Can you work these out from the model? Positions are in its coordinate system, mm. A direction names the side the tool comes from. Round coordinates to 2 decimals unless told otherwise and drop trailing zeros. Loops run counter-clockwise (first coordinate to the right, second up) from the corner with the lowest first, then second, coordinate; pieces in that order, holes last. Notation, with made-up numbers: M 75.25,17 L 111.25,17 A17 cw 111.25,43 Z; hole C 70.5,42.25 d7. An arc over 180 degrees is marked long. Answer as CSV lines item,"result".
from build123d import *

# Parameters (mm, degrees)
BOSS_EXTRUDE1_DEPTH     = 6
CUT_EXTRUDE1_DEPTH      = 33.32645975048922
CUT_EXTRUDE1_DEPTH_BACK = 33.32645975048922
SKETCH3_R               = 1.7500000000000002
SKETCH3_R_2             = 1.7499999999999998
SKETCH6_R               = 3.2500000000000004
SKETCH6_R_2             = 3.25
CUT_EXTRUDE2_DEPTH      = 3.5
SKETCH7_W               = 11.699999999999998
SKETCH7_H               = 27.786688839798195
BOSS_EXTRUDE2_DEPTH     = 6
SKETCH8_W               = 11.699999999999998
SKETCH8_H               = 27.786688839798195
CUT_EXTRUDE3_DEPTH      = 2
FILLET1_R               = 2
FILLET2_R               = 2
FILLET3_R               = 2
CUT_EXTRUDE4_DEPTH      = 52.48495646180262
CUT_EXTRUDE4_DEPTH_BACK = 52.48495646180262
CUT_EXTRUDE5_DEPTH      = 52.48495646180262
CUT_EXTRUDE5_DEPTH_BACK = 2
FILLET4_R               = 2
FILLET5_R               = 2


with BuildPart() as part:
    # Sketch2 → Boss-Extrude1 (new body)
    with BuildSketch(Plane.XY):
        Polygon((-27.999999999999996, 15), (1.84e-15, 15), (0, 0), (-27.999999999999996, 0), align=None)
    extrude(amount=BOSS_EXTRUDE1_DEPTH)

    # Sketch3 → Cut-Extrude1 (cut, two sides: drawn at the far end of the back side and taken through both)
    with BuildSketch(Plane.XY.offset(6).offset(-CUT_EXTRUDE1_DEPTH_BACK)):
        with Locations((-21.5, 4.999999999999999)):
            Circle(SKETCH3_R)
        with Locations((-6.5, 4.999999999999999)):
            Circle(SKETCH3_R_2)
    extrude(amount=CUT_EXTRUDE1_DEPTH + CUT_EXTRUDE1_DEPTH_BACK, mode=Mode.SUBTRACT)

    # Sketch6 → Cut-Extrude2 (cut)
    with BuildSketch(Plane.XY.offset(6)):
        with Locations((-21.5, 4.999999999999999)):
            Circle(SKETCH6_R)
        with Locations((-6.500000000000001, 4.999999999999999)):
            Circle(SKETCH6_R_2)
    extrude(amount=-CUT_EXTRUDE2_DEPTH, mode=Mode.SUBTRACT)

    # Sketch7 → Boss-Extrude2 (add)
    with BuildSketch(Plane(origin=(0, 0, 0), x_dir=(-1, 0, 0), z_dir=(0, 0, -1))):
        with Locations((14, 28.893344419899098)):
            Rectangle(SKETCH7_W, SKETCH7_H)
    extrude(amount=-BOSS_EXTRUDE2_DEPTH)

    # Sketch8 → Cut-Extrude3 (cut)
    with BuildSketch(Plane(origin=(0, 0, 0), x_dir=(-1, 0, 0), z_dir=(0, 0, -1))):
        with Locations((14, 28.893344419899098)):
            Rectangle(SKETCH8_W, SKETCH8_H)
    extrude(amount=-CUT_EXTRUDE3_DEPTH, mode=Mode.SUBTRACT)

    # Fillet1
    fillet1_edges = [part.edges().sort_by_distance(p)[0] for p in [
        (-14, 15, 2),
    ]]
    fillet(fillet1_edges, radius=FILLET1_R - 0.0001)  # a hair under: the kernel refuses the full size

    # Fillet2
    fillet2_edges = [part.edges().sort_by_distance(p)[0] for p in [
        (-8.15, 15, 3.0000500000000003),
    ]]
    fillet(fillet2_edges, radius=FILLET2_R)

    # Fillet3
    fillet3_edges = [part.edges().sort_by_distance(p)[0] for p in [
        (-19.849999999999998, 15, 3.00005),
    ]]
    fillet(fillet3_edges, radius=FILLET3_R)

    # Sketch9 → Cut-Extrude4 (cut, two sides: drawn at the far end of the back side and taken through both)
    with BuildSketch(Plane.XY.offset(6).offset(-CUT_EXTRUDE4_DEPTH_BACK)):
        with BuildLine():
            Line((-12.28493666219322, 38.78668883979819), (-12.284936662193216, 18.786688839798188))
            ThreePointArc((-12.284936662193216, 18.786688839798188), (-14.034936662193216, 17.036688839798188), (-15.784936662193216, 18.786688839798188))
            Line((-15.784936662193216, 18.786688839798188), (-15.78493666219322, 38.78668883979819))
            ThreePointArc((-15.78493666219322, 38.78668883979819), (-14.03493666219322, 40.53668883979819), (-12.28493666219322, 38.78668883979819))
        make_face()
    extrude(amount=CUT_EXTRUDE4_DEPTH + CUT_EXTRUDE4_DEPTH_BACK, mode=Mode.SUBTRACT)

    # Sketch10 → Cut-Extrude5 (cut, two sides: drawn at the far end of the back side and taken through both)
    with BuildSketch(Plane.XY.offset(6).offset(-CUT_EXTRUDE5_DEPTH_BACK)):
        with BuildLine():
            Line((-10.784936662193223, 38.78668883979819), (-10.78493666219322, 18.786688839798188))
            ThreePointArc((-10.78493666219322, 18.786688839798188), (-14.034936662193216, 15.536688839798186), (-17.284936662193218, 18.786688839798188))
            Line((-17.284936662193218, 18.786688839798188), (-17.284936662193218, 38.78668883979819))
            ThreePointArc((-17.284936662193218, 38.78668883979819), (-14.03493666219322, 42.03668883979819), (-10.784936662193223, 38.78668883979819))
        make_face()
    extrude(amount=CUT_EXTRUDE5_DEPTH + CUT_EXTRUDE5_DEPTH_BACK, mode=Mode.SUBTRACT)

    # Fillet4
    fillet4_edges = [part.edges().sort_by_distance(p)[0] for p in [
        (-8.15, 42.786688839798195, 4),
        (-19.849999999999998, 42.786688839798195, 4),
    ]]
    fillet(fillet4_edges, radius=FILLET4_R)

    # Fillet5
    fillet5_edges = [part.edges().sort_by_distance(p)[0] for p in [
        (-27.999999999999996, 15, 3),
        (1.84e-15, 15, 3),
    ]]
    fillet(fillet5_edges, radius=FILLET5_R)


solid = part.part
Item 1: If we section it at D-D on z = 1: Write out the boundary of the cut face in (x, y), then the cut area to 3 significant figures.
Output:
outline,"M -28,0 L 0,0 L 0,13 A2 ccw -2,15 L -6.15,15 A2 cw -7.15,15.27 L -20.85,15.27 A2 cw -21.85,15 L -26,15 A2 ccw -28,13 Z; hole C -21.5,5 d3.5; hole C -6.5,5 d3.5"
area,"403 mm2"
Item 2: On a 3-axis mill with a long thin cutter (end or side, diameter ignored), from which of +Z, -Z, +X, -X, +Y, -Y can I reach the whole of each face in a straight line? I mean faces 1 (the face through (-8.895, 7.197, 4.274)), 2 (the face through (0, 7, 3)), 3 (the face through (-12.285, 29, 3)). Say none if no direction works.
Output:
face 1,"+Z"
face 2,"+Z, -Z, +X, +Y, -Y"
face 3,"+Z, -Z"
Item 3: If we section it at A-A on y = 36.5: Write out the boundary of the cut face in (x, z), then the cut area to 3 significant figures.
Output:
outline,"M -19.85,2 L -15.78,2 L -15.78,4 L -17.28,4 L -17.28,6 L -19.85,6 Z; M -12.28,2 L -8.15,2 L -8.15,6 L -10.78,6 L -10.78,4 L -12.28,4 Z"
area,"26.8 mm2"
Item 4: If I drill on line 1 along X through (y, z) = (5, 1.1); line 2 along X through (y, z) = (27, 2.75); line 3 along Z through (x, y) = (-13.25, 17), over which ranges is the centre line in solid material (lowest first)? Write a range as from..to.
Output:
line 1,"x = -28..-23.25, -19.75..-8.25, -4.75..0"
line 2,"x = -19.85..-15.78, -12.28..-8.15"
line 3,"z = 2..4"
Item 5: We'd pull the mould along X, two halves only. Please class faces 4 (the face through (-6.88, 3.29, 1.23)), 5 (the face through (-8.15, 29, 4)), 6 (the face through (-6, 15, 3)): released by +X, released by -X, zero draft, split by the parting line, or undercut.
Output:
face 4,"undercut"
face 5,"released by +X"
face 6,"zero draft"
Item 6: Will these pins go through, and if not, where does the flat tip stop? pin 1 (2 mm diameter, centred on y = 25, z = 3, fed in from -X); pin 2 (4.5 mm diameter, centred on x = -21.5, y = 5, fed in from +Z); pin 3 (13 mm diameter, centred on x = -14.5, y = 34, fed in from -Z).
Output:
pin 1,"stops at x = -19.85"
pin 2,"stops at z = 2.5"
pin 3,"stops at z = 2"
Item 7: If we section it at C-C on y = 5: Write out the boundary of the cut face in (x, z).
Output:
outline,"M -28,0 L -23.25,0 L -23.25,2.5 L -24.75,2.5 L -24.75,6 L -28,6 Z; M -19.75,0 L -8.25,0 L -8.25,2.5 L -9.75,2.5 L -9.75,6 L -18.25,6 L -18.25,2.5 L -19.75,2.5 Z; M -4.75,0 L 0,0 L 0,6 L -3.25,6 L -3.25,2.5 L -4.75,2.5 Z"
Item 8: If we section it at B-B on z = 5: Write out the boundary of the cut face in (x, y).
Output:
outline,"M -28,0 L 0,0 L 0,13 A2 ccw -2,15 L -6.15,15 A2 cw -8.15,17 L -8.15,40.79 A2 ccw -10.15,42.79 L -17.85,42.79 A2 ccw -19.85,40.79 L -19.85,17 A2 cw -21.85,15 L -26,15 A2 ccw -28,13 Z; hole C -21.5,5 d6.5; hole M -17.28,18.79 A3.25 ccw -10.78,18.79 L -10.78,38.79 A3.25 ccw -17.28,38.79 Z; hole C -6.5,5 d6.5"
